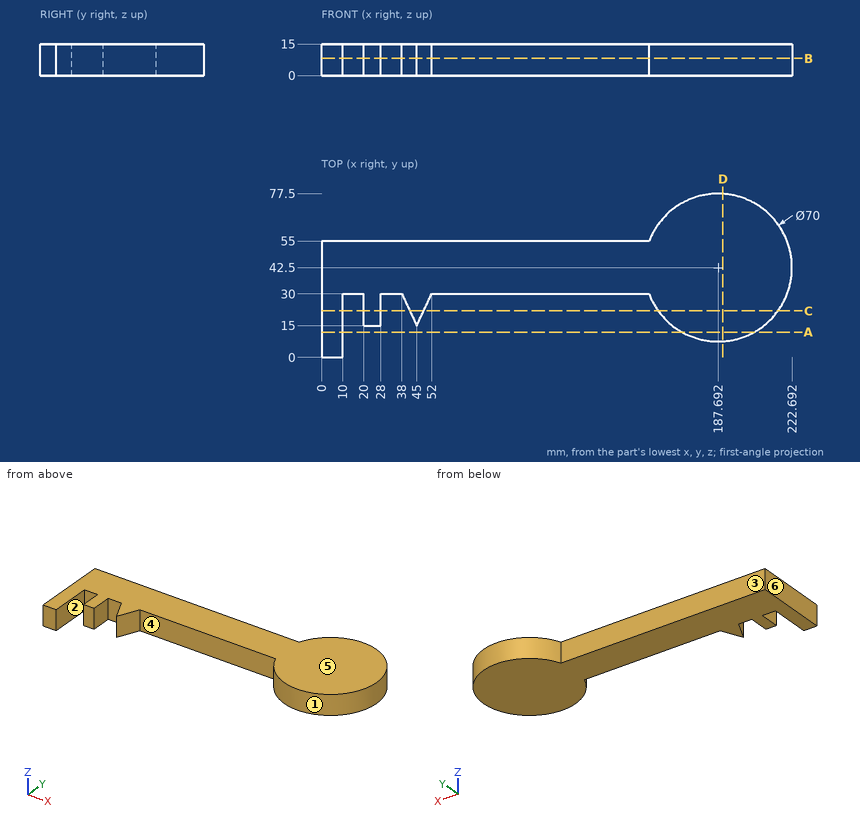
Geometry: see drawing. Coordinates: mm, zero at the bounding-box minimum. A direction names the side the tool comes from. Round coordinates to 2 decimals unless told otherwise and drop trailing zeros. Loops run counter-clockwise (first coordinate to the right, second up) from the corner with the lowest first, then second, coordinate; pieces in that order, holes last. Notation, with made-up numbers: M 67,-12.75 L 90,-12.75 A31 cw 90,24.25 Z; hole C -16.5,76 d9. An arc over 180 degrees is marked long. Use a Markdown table: item, result. Add a question column.
1. Ray query, line 1 along X through (y, z) = (17.5, 3.5); line 2 along Y through (x, z) = (106, 14.75); line 3 along Y through (x, z) = (22, 7). Return the intervals inside material, ascending. Write a range as [from, to].
2. Cut plane A-A, the plane y = 12. Output: boundary loops of the cut face in (x, z).
3. Contact query for flat-ended pins moving along their axis: pin 1 (7.5 mm diameter, centred on y = 19, z = 7.5, fed in from +X); pin 2 (1.5 mm diameter, centred on x = 110, z = 7.5, fed in from +Y); pin 3 (4.5 mm diameter, centred on y = 8.5, z = 6, fed in from +X). Output: stop coordinate, or through.
4. Pull-direction query (X, two-part tool) for the marked faces 4, 5 and 6; classes: +X half, -X half, draft (parallel to the pull), parting line (faces both ways), or undercut.
5. Set-up query: the marked faces 1, 2 and 3. Return all of +Z, -Z, +X, -X, +Y, -Y with unobstructed straight access to the full face (end or side cutting, diameter ignored); none if empty.
6. Cut plane D-D, the plane x = 190. Output: boundary loops of the cut face in (y, z).
7. Cut plane C-C, the plane y = 22. Output: boundary loops of the cut face in (x, z), and give its area (3 significant figures).
8. Cut plane B-B, the plane z = 8.25. Output: boundary loops of the cut face in (x, y).
Solution:
| question | item | result |
|---|---|---|
| 1 | line 1 | x = [0, 10], [20, 28], [43.83, 46.17], [163.2, 212.19] |
| 1 | line 2 | y = [30, 55] |
| 1 | line 3 | y = [15, 55] |
| 2 | outline | M 0,0 L 10,0 L 10,15 L 0,15 Z; M 170.52,0 L 204.86,0 L 204.86,15 L 170.52,15 Z |
| 3 | pin 1 | stops at x = 216.59 |
| 3 | pin 2 | stops at y = 55 |
| 3 | pin 3 | stops at x = 202.42 |
| 4 | face 4 | undercut |
| 4 | face 5 | draft |
| 4 | face 6 | -X half |
| 5 | face 1 | +Z, -Z |
| 5 | face 2 | +Z, -Z, -Y |
| 5 | face 3 | +Z, -Z, -X, +Y |
| 6 | outline | M 7.58,0 L 77.42,0 L 77.42,15 L 7.58,15 Z |
| 7 | outline | M 0,0 L 10,0 L 10,15 L 0,15 Z; M 20,0 L 28,0 L 28,15 L 20,15 Z; M 41.73,0 L 48.27,0 L 48.27,15 L 41.73,15 Z; M 159.32,0 L 216.06,0 L 216.06,15 L 159.32,15 Z |
| 7 | area | 1,220 mm2 |
| 8 | outline | M 0,0 L 10,0 L 10,30 L 20,30 L 20,15 L 28,15 L 28,30 L 38,30 L 45,15 L 52,30 L 155,30 A35 ccw long 155,55 L 0,55 Z |
